```python
from build123d import *

# Parameters (mm, degrees)
SKETCH_1_W             = 23.5
SKETCH_1_H             = 12
EXTRUDE_1_DEPTH        = 650.5
HOLE_WIZARD_M6_1_D     = 5
HOLE_WIZARD_M6_1_DEPTH = 19
HOLE_WIZARD_M6_1_TIP   = 1.502151548
HOLE_WIZARD_M6_2_D     = 5
HOLE_WIZARD_M6_2_DEPTH = 19
HOLE_WIZARD_M6_2_TIP   = 1.502151548
HOLE_WIZARD_M4_1_D     = 3.3
HOLE_WIZARD_M4_1_DEPTH = 15
HOLE_WIZARD_M4_1_TIP   = 0.991420021


with BuildPart() as part:
    # 草图1 → 凸台-拉伸1 (new, symmetric)
    with BuildSketch(Plane(origin=(0, 0, 0), x_dir=(0, 0, -1), z_dir=(1, 0, 0))):
        Polygon((-15, 15), (-11.5, 15), (-11.5, 13.5), (-11, 13.5), (-11, 12), (-9.5, 12), (-9.5, 15), (-8, 15), (-8, 12.5), (-5, 12.5), (-5, 15), (5, 15), (5, 12.5), (8, 12.5), (8, 15), (9.5, 15), (9.5, 12), (11, 12), (11, 13.5), (11.5, 13.5), (11.5, 15), (15, 15), (15, 8), (12.5, 8), (12.5, 5), (15, 5), (15, -5), (12.5, -5), (12.5, -8), (15, -8), (15, -15), (11.5, -15), (11.5, -13.5), (11, -13.5), (11, -12), (9.5, -12), (9.5, -15), (8, -15), (8, -12.5), (5, -12.5), (5, -15), (-5, -15), (-5, -12.5), (-8, -12.5), (-8, -15), (-9.5, -15), (-9.5, -12), (-11, -12), (-11, -13.5), (-11.5, -13.5), (-11.5, -15), (-15, -15), align=None)
        with BuildLine():
            Line((12, -10.5), (12, -8.5))
            ThreePointArc((12, -8.5), (11.853553391, -8.146446609), (11.5, -8))
            Line((11.5, -8), (-11.5, -8))
            ThreePointArc((-11.5, -8), (-11.853553391, -8.146446609), (-12, -8.5))
            Line((-12, -8.5), (-12, -10.5))
            ThreePointArc((-12, -10.5), (-11.853553391, -10.853553391), (-11.5, -11))
            Line((-11.5, -11), (11.5, -11))
            ThreePointArc((11.5, -11), (11.853553391, -10.853553391), (12, -10.5))
        make_face(mode=Mode.SUBTRACT)
        with BuildLine():
            Line((-11.5, 11), (11.5, 11))
            ThreePointArc((11.5, 11), (11.853553391, 10.853553391), (12, 10.5))
            Line((12, 10.5), (12, 8.5))
            ThreePointArc((12, 8.5), (11.853553391, 8.146446609), (11.5, 8))
            Line((11.5, 8), (-11.5, 8))
            ThreePointArc((-11.5, 8), (-11.853553391, 8.146446609), (-12, 8.5))
            Line((-12, 8.5), (-12, 10.5))
            ThreePointArc((-12, 10.5), (-11.853553391, 10.853553391), (-11.5, 11))
        make_face(mode=Mode.SUBTRACT)
        Rectangle(SKETCH_1_W, SKETCH_1_H, mode=Mode.SUBTRACT)
    extrude(amount=EXTRUDE_1_DEPTH, both=True)

    # M6 螺纹孔1
    with Locations(Plane(origin=(0, -15, 0), x_dir=(-1, 0, 0), z_dir=(0, -1, 0))):
        with Locations((615.5, 0), (630.5, 0), (-615.5, 0), (-630.5, 0)):
            Hole(HOLE_WIZARD_M6_1_D / 2, depth=HOLE_WIZARD_M6_1_DEPTH)
            with Locations((0, 0, -(HOLE_WIZARD_M6_1_DEPTH + HOLE_WIZARD_M6_1_TIP / 2))):  # 118° drill point
                Cone(0, HOLE_WIZARD_M6_1_D / 2, HOLE_WIZARD_M6_1_TIP, mode=Mode.SUBTRACT)

    # M6 螺纹孔2
    with Locations(Plane(origin=(0, 0, -15), x_dir=(-1, 0, 0), z_dir=(0, 0, -1))):
        with Locations((-630.5, 0), (-615.5, 0), (630.5, 0), (615.5, 0)):
            Hole(HOLE_WIZARD_M6_2_D / 2, depth=HOLE_WIZARD_M6_2_DEPTH)
            with Locations((0, 0, -(HOLE_WIZARD_M6_2_DEPTH + HOLE_WIZARD_M6_2_TIP / 2))):  # 118° drill point
                Cone(0, HOLE_WIZARD_M6_2_D / 2, HOLE_WIZARD_M6_2_TIP, mode=Mode.SUBTRACT)

    # M4 螺纹孔1
    with Locations(Plane(origin=(0, 0, -15), x_dir=(-1, 0, 0), z_dir=(0, 0, -1))):
        with Locations((560, 0), (280, 0), (0, 0), (-280, 0), (-560, 0)):
            Hole(HOLE_WIZARD_M4_1_D / 2, depth=HOLE_WIZARD_M4_1_DEPTH)
            with Locations((0, 0, -(HOLE_WIZARD_M4_1_DEPTH + HOLE_WIZARD_M4_1_TIP / 2))):  # 118° drill point
                Cone(0, HOLE_WIZARD_M4_1_D / 2, HOLE_WIZARD_M4_1_TIP, mode=Mode.SUBTRACT)


solid = part.part
```
Input: part model. Units: mm. Frame: model coordinates. A direction names the side the tool comes from. Coordinates: 2 decimals unless noted, no trailing zeros. Put each result on its own line as item: value. Start each with the question number.
1) Ray query, L1, parallel to Y at x = 364.5, z = -8.25; L2, parallel to Y at x = -280, z = -13.3; L3, parallel to Z at x = 35, y = -2.75. Return the intervals inside material, ascending.
2) Mould query, pull axis Z, two halves, no side actions, for faces 3 (the face through (650.5, 7, 0)), 4 (the face through (9, 6, 0)), 5 (the face through (9, 0, 15)). Classes: pulls with the +Z half, pulls with the -Z half, needs draft (parallel to the pull), parting line crosses it, or undercut.
3) Contact query for flat-ended pins moving along their axis: pin 1 (3 mm diameter, centred on x = -438.5, z = -6, fed in from -Y); pin 2 (1.5 mm diameter, centred on x = 315.5, y = 7, fed in from -Z); pin 3 (4.5 mm diameter, centred on x = 630.5, z = 0, fed in from -Y); pin 4 (4.5 mm diameter, centred on x = 615.5, y = 0, fed in from -Z). Output: stop coordinate, or through.
4) Cut plane A-A (x = 356.5). State how many separate pieces and enclosed holes the cut face has, plus the area to 3 significant figures.
5) Reachability of faces 1 (the face through (-650.5, 7, 0)), 2 (the face through (9, -8, 0)) from +Z, -Z, +X, -X, +Y, -Y: full face, straight path, thin tool, end or side. Return the list, or none.
Resolved:
1. L1: y = -15 to -11, -8 to -6, 6 to 8, 11 to 15
1. L2: y = -15 to -8, -5 to -1.65, 1.65 to 5, 8 to 15
1. L3: z = -15 to -11.75, 11.75 to 15
2. face 3: needs draft
2. face 4: undercut
2. face 5: pulls with the +Z half
3. pin 1: stops at y = -15
3. pin 2: stops at z = -12.5
3. pin 3: stops at y = 6
3. pin 4: stops at z = 11.75
4. separate pieces: 1
4. enclosed holes: 3
4. area: 408 mm2
5. face 1: +Z, -Z, -X, +Y, -Y
5. face 2: +X, -X
